from build123d import *

# Parameters (mm, degrees)
BOSS_EXTRUDE1_DEPTH = 2
SKETCH5_W           = 18
SKETCH5_H           = 2
BOSS_EXTRUDE2_DEPTH = 5
CUT_EXTRUDE1_REACH  = 4
SKETCH6_R           = 1.6
FILLET1_R           = 2.5
SKETCH7_W           = 18
SKETCH7_H           = 0.9
BOSS_EXTRUDE3_DEPTH = 1


with BuildPart() as part:
    # Sketch4 → Boss-Extrude1 (new body)
    with BuildSketch(Plane(origin=(0, 0, 0), x_dir=(1, 0, 0), z_dir=(0, 1, 0))):
        Polygon((-56.8, -3.5), (-56.8, 105.1), (3.5, 105.1), (3.5, -3.5), (-2.3, -3.5), (-14.3, -3.5), (-30.8, -3.5), (-45.8, -3.5), align=None)
    extrude(amount=BOSS_EXTRUDE1_DEPTH)

    # Sketch5 → Boss-Extrude2 (add)
    with BuildSketch(Plane(origin=(0, 2, 0), x_dir=(1, 0, 0), z_dir=(0, 1, 0))):
        Polygon((-45.3, -1.5), (-54.8, -1.5), (-54.8, 103.1), (1.5, 103.1), (1.5, -1.5), (-3.3, -1.5), (-3.3, -3.5), (3.5, -3.5), (3.5, 105.1), (-56.8, 105.1), (-56.8, -3.5), (-45.3, -3.5), align=None)
        with Locations((-22.3, -2.5)):
            Rectangle(SKETCH5_W, SKETCH5_H)
    extrude(amount=BOSS_EXTRUDE2_DEPTH)

    # Sketch6 → Cut-Extrude1 (cut, up to next)
    with BuildSketch(Plane(origin=(0, 2, 0), x_dir=(1, 0, 0), z_dir=(0, 1, 0)), mode=Mode.PRIVATE) as cut_extrude1_sk1:
        with Locations((-2.5, 96.52)):
            Circle(SKETCH6_R)
    cut_extrude1_tool1 = extrude(cut_extrude1_sk1.sketch, amount=-CUT_EXTRUDE1_REACH, mode=Mode.PRIVATE) & part.part
    add(cut_extrude1_tool1.solids().sort_by_distance((-2.5, 2, -96.52))[0], mode=Mode.SUBTRACT)
    # Sketch6 → Cut-Extrude1 (cut, up to next)
    with BuildSketch(Plane(origin=(0, 2, 0), x_dir=(1, 0, 0), z_dir=(0, 1, 0)), mode=Mode.PRIVATE) as cut_extrude1_sk2:
        with Locations((-50.7, 89.7)):
            Circle(SKETCH6_R)
    cut_extrude1_tool2 = extrude(cut_extrude1_sk2.sketch, amount=-CUT_EXTRUDE1_REACH, mode=Mode.PRIVATE) & part.part
    add(cut_extrude1_tool2.solids().sort_by_distance((-50.7, 2, -89.7))[0], mode=Mode.SUBTRACT)
    # Sketch6 → Cut-Extrude1 (cut, up to next)
    with BuildSketch(Plane(origin=(0, 2, 0), x_dir=(1, 0, 0), z_dir=(0, 1, 0)), mode=Mode.PRIVATE) as cut_extrude1_sk3:
        with Locations((-2.5, 13.5)):
            Circle(SKETCH6_R)
    cut_extrude1_tool3 = extrude(cut_extrude1_sk3.sketch, amount=-CUT_EXTRUDE1_REACH, mode=Mode.PRIVATE) & part.part
    add(cut_extrude1_tool3.solids().sort_by_distance((-2.5, 2, -13.5))[0], mode=Mode.SUBTRACT)
    # Sketch6 → Cut-Extrude1 (cut, up to next)
    with BuildSketch(Plane(origin=(0, 2, 0), x_dir=(1, 0, 0), z_dir=(0, 1, 0)), mode=Mode.PRIVATE) as cut_extrude1_sk4:
        with Locations((-50.7, 14.8)):
            Circle(SKETCH6_R)
    cut_extrude1_tool4 = extrude(cut_extrude1_sk4.sketch, amount=-CUT_EXTRUDE1_REACH, mode=Mode.PRIVATE) & part.part
    add(cut_extrude1_tool4.solids().sort_by_distance((-50.7, 2, -14.8))[0], mode=Mode.SUBTRACT)

    # Fillet1
    fillet1_edges = [part.edges().sort_by_distance(p)[0] for p in [
        (3.5, 3.5, 3.5),
        (3.5, 3.5, -105.1),
        (-56.8, 3.5, -105.1),
        (-56.8, 3.5, 3.5),
        (1.5, 4.5, 1.5),
        (-54.8, 4.5, 1.5),
        (-54.8, 4.5, -103.1),
        (1.5, 4.5, -103.1),
    ]]
    fillet(fillet1_edges, radius=FILLET1_R)

    # Sketch7 → Boss-Extrude3 (add)
    with BuildSketch(Plane(origin=(0, 7, 0), x_dir=(1, 0, 0), z_dir=(0, 1, 0))):
        with BuildLine():
            Line((-3.3, -2.4), (-1, -2.4))
            ThreePointArc((-1, -2.4), (1.404163056, -1.404163056), (2.4, 1))
            Line((2.4, 1), (2.4, 100.6))
            ThreePointArc((2.4, 100.6), (1.404163056, 103.004163056), (-1, 104))
            Line((-1, 104), (-52.3, 104))
            ThreePointArc((-52.3, 104), (-54.704163056, 103.004163056), (-55.7, 100.6))
            Line((-55.7, 100.6), (-55.7, 1))
            ThreePointArc((-55.7, 1), (-54.704163056, -1.404163056), (-52.3, -2.4))
            Line((-52.3, -2.4), (-45.3, -2.4))
            Line((-45.3, -2.4), (-45.3, -1.5))
            Line((-45.3, -1.5), (-52.3, -1.5))
            ThreePointArc((-52.3, -1.5), (-54.067766953, -0.767766953), (-54.8, 1))
            Line((-54.8, 1), (-54.8, 100.6))
            ThreePointArc((-54.8, 100.6), (-54.067766953, 102.367766953), (-52.3, 103.1))
            Line((-52.3, 103.1), (-1, 103.1))
            ThreePointArc((-1, 103.1), (0.767766953, 102.367766953), (1.5, 100.6))
            Line((1.5, 100.6), (1.5, 1))
            ThreePointArc((1.5, 1), (0.767766953, -0.767766953), (-1, -1.5))
            Line((-1, -1.5), (-3.3, -1.5))
            Line((-3.3, -1.5), (-3.3, -2.4))
        make_face()
        with Locations((-22.3, -1.95)):
            Rectangle(SKETCH7_W, SKETCH7_H)
    extrude(amount=BOSS_EXTRUDE3_DEPTH)


solid = part.part
The listing builds one solid part. Answer for the finished solid, in the listing's coordinates (mm). A direction names the side the tool comes from. Give positions to 0.01 mm unless a question says otherwise; leave off trailing zeros. Loops run counter-clockwise (first coordinate to the right, second up) from the corner with the lowest first, then second, coordinate; pieces in that order, holes last.
Item 1: Each of these flat-tipped pins is pushed along its axis until it touches: pin 1 Ø0.9 at (x, z) = (-24.5, 3) entering from +Y; pin 2 Ø3 at (x, z) = (-50.7, -89.7) entering from -Y (3 decimals); pin 3 Ø4 at (x, z) = (-2.5, -13.5) entering from +Y; pin 4 Ø0.5 at (y, z) = (7.5, -48.5) entering from -X. Where does it stop, or does it pass through?
Derived:
pin 1: stops at y = 7
pin 2: passes through
pin 3: stops at y = 2
pin 4: stops at x = -55.7
Item 2: A tool of negligible diameter and unlimited length cuts with its end or side. For faces 1 (the cylindrical face through (-49.84, 1.01, -91.05)), 2 (the cylindrical face through (-54.68, 7.49, -103.03)), 3 (the flat face through (-49, 5, 1.5)), 4 (the cylindrical face through (1.38, 7.49, 1.43)), 5 (the flat face through (-3.3, 5, 2)), from which of +Z, -Z, +X, -X, +Y, -Y can it reach the whole face along a straight path? Write none if from no direction.
Derived:
face 1: +Y, -Y
face 2: -Z, -X, +Y
face 3: +Y
face 4: +Z, +X, +Y
face 5: +Z, +Y
Item 3: A cutting plane is placed at A-A (y = 4). Give the vertices of the cut face in (x, z).
Derived:
outline: (-56.8, -102.6) arc R2.5 ccw to (-54.3, -105.1) - (1, -105.1) arc R2.5 ccw to (3.5, -102.6) - (3.5, 1) arc R2.5 ccw to (1, 3.5) - (-3.3, 3.5) - (-3.3, 1.5) - (-1, 1.5) arc R2.5 cw to (1.5, -1) - (1.5, -100.6) arc R2.5 cw to (-1, -103.1) - (-52.3, -103.1) arc R2.5 cw to (-54.8, -100.6) - (-54.8, -1) arc R2.5 cw to (-52.3, 1.5) - (-45.3, 1.5) - (-45.3, 3.5) - (-54.3, 3.5) arc R2.5 ccw to (-56.8, 1) - close; (-31.3, 1.5) - (-13.3, 1.5) - (-13.3, 3.5) - (-31.3, 3.5) - close
Item 4: Determine the mould class of faces 6 (the flat face through (-26, 2, -51)), 7 (the cylindrical face through (-54.73, 7.49, 1.38)), 8 (the flat face through (-26, 3, -105.1)) for opening direction Z: +Z half, -Z half, draft (parallel to the pull), parting line (faces both ways), or undercut.
Derived:
face 6: undercut
face 7: +Z half
face 8: -Z half
Item 5: Find the intervals of material crossed by line 1 along Z through (x, y) = (-2.5, 1.05); line 2 along Z through (x, y) = (-50.7, 0.7); line 3 along X through (y, z) = (0.8, -13.5), in increasing order.
Derived:
line 1: z = -105.1 to -98.12, -94.92 to -15.1, -11.9 to 3.5
line 2: z = -105.1 to -91.3, -88.1 to -16.4, -13.2 to 3.5
line 3: x = -56.8 to -51.63, -49.77 to -4.1, -0.9 to 3.5
Item 6: A cutting plane is placed at B-B (x = -50.7). Give the vertices of the cut face in (y, z).
Derived:
outline: (0, -105.1) - (7, -105.1) - (7, -104) - (8, -104) - (8, -103.1) - (2, -103.1) - (2, -91.3) - (0, -91.3) - close; (0, -88.1) - (2, -88.1) - (2, -16.4) - (0, -16.4) - close; (0, -13.2) - (2, -13.2) - (2, 1.5) - (8, 1.5) - (8, 2.4) - (7, 2.4) - (7, 3.5) - (0, 3.5) - close
Item 7: A cutting plane is placed at C-C (z = -96.52). Give the vertices of the cut face in (x, y), then the cut area to 3 significant figures.
Derived:
outline: (-56.8, 0) - (-4.1, 0) - (-4.1, 2) - (-54.8, 2) - (-54.8, 8) - (-55.7, 8) - (-55.7, 7) - (-56.8, 7) - close; (-0.9, 0) - (3.5, 0) - (3.5, 7) - (2.4, 7) - (2.4, 8) - (1.5, 8) - (1.5, 2) - (-0.9, 2) - close
area: 136 mm2
Item 8: A cutting plane is placed at D-D (x = -33). Give the vertices of the cut face in (y, z).
Derived:
outline: (0, -105.1) - (7, -105.1) - (7, -104) - (8, -104) - (8, -103.1) - (2, -103.1) - (2, 3.5) - (0, 3.5) - close
